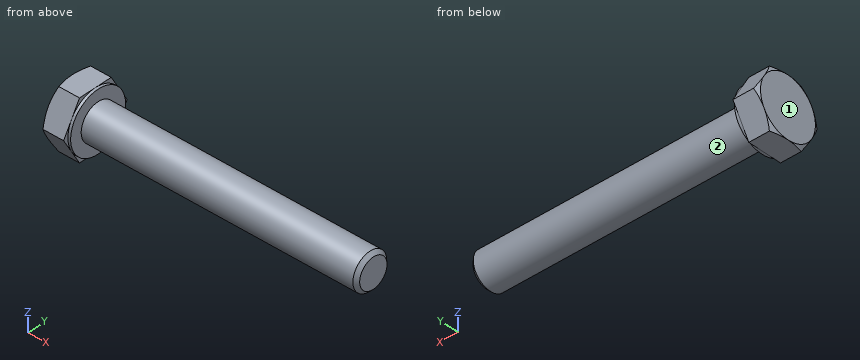
Autodesk Inventor part; units mm, degrees
ref_plane "Work Plane1" through (1.525, 0, 0) normal (0, 0, 1) x (1, 0, 0)
ref_plane "YZ Plane" through (0, 0, 0) normal (1, 0, 0) x (0, 1, 0)
ref_plane "XZ Plane" through (0, 0, 0) normal (0, 1, 0) x (-1, 0, 0)
sketch "Sketch1" plane through (0, 0, 0) normal (0, 0, 1) x (1, 0, 0)
  line L0 (0, 6.5) -> (0, 4)
  line L1 (38, 4) -> (60, 4)
  line L2 (60, 4) -> (60, 0)
  line L3 (60, 0) -> (-0.6001, 0)
  line L4 (-12.7201, 0) -> (72.12, 0)
  line L5 (-0.6001, 0) -> (-0.6001, 6.5)
  line L6 (-0.6001, 6.5) -> (0, 6.5)
  line L7 (38, 4) -> (37.2331, 4)
  line L8 (37.2331, 4) -> (0, 4)
  line L9 (0, -1.3) -> (0, 7.8)
  dimension "d0" = 60
  dimension "d1" = 22
  dimension "d2" = 8
  dimension "d9" = 0.6001
  dimension "d10" = 13
  dimension "d13" = 0.7669
  dimension "d14" = 8
revolve "Body" add sketch "Sketch1" angle 360 about axis through (60, 0, 0) along (-1, 0, 0)
sketch "Sketch2" plane through (-0.6001, 0, 0) normal (-1, 0, 0) x (0, 0, 1)
  line L0 (0, 7.5056) -> (6.5, 3.7528)
  line L1 (6.5, 3.7528) -> (6.5, -3.7528)
  line L2 (6.5, -3.7528) -> (0, -7.5056)
  line L3 (0, -7.5056) -> (-6.5, -3.7528)
  line L4 (-6.5, -3.7528) -> (-6.5, 3.7528)
  line L5 (-6.5, 3.7528) -> (0, 7.5056)
  point P0 (0, 0)
  point P1 (0, 0)
  dimension "d11" = 13
extrude "Head" add sketch "Sketch2" along normal blind 5.08
sketch "Sketch4" plane through (0, 0, 0) normal (0, 0, 1) x (1, 0, 0)
  line L0 (-5.6801, 6.5) -> (-5.6801, 7.5056)
  line L1 (-5.6801, 7.5056) -> (-5.0995, 7.5056)
  line L2 (-5.0995, 7.5056) -> (-5.6801, 6.5)
  line L3 (-6.6961, 0) -> (0.4159, 0)
  line L4 (-0.6001, 7.5056) -> (-5.6801, 7.5056)
  line L5 (-5.6801, 3.7528) -> (-5.6801, 7.5056)
  dimension "d5" = 30
  dimension "d19" = 13
revolve "Chamfer1" cut sketch "Sketch4" angle 360 about axis through (-10, 0, 0) along (1, 0, 0)
thread "Thread"
chamfer "Chamfer2" distance 0.7668 distance2 0.7669 1 edges at (60, -4, 0) measured on face at (60, -0.1514, -1.2467)
ref_plane "Work Plane1" through (1.525, 0, 0) normal (0, 0, 1) x (1, 0, 0)
equation "\"d0\" = NLG"
equation "\"d1\" = GEL"
equation "\"d2\" = GD"
equation "\"d10\" = SD2"
equation "\"d14\" = BDM"
equation "\"d11\" = SW"
equation "\"d3\" = KOH - SD"
equation "\"d5\" = ANG1"
equation "\"d19\" = SW0"
equation "\"d15\" = GEL"
equation "\"d6\" = -0.5 * SPD + 0.5 * GD"
equation "\"NLG\" = 60"
equation "\"GD\" = NND"
equation "\"BDM\" = NND"
equation "\"KOH\" = 5.68"
equation "\"GEL\" = 22"
equation "\"SW\" = 13"
equation "\"SW0\" = SW"
equation "\"SPD\" = NND - 1.2269 * PTC"
equation "\"SD2\" = SW"
equation "\"SD\" = 0.6"
equation "\"ANG1\" = 30deg"
equation "\"GAL\" = 0.61345 * PTC"
equation "\"GUL\" = 0.61345 * PTC"
equation "\"RR\" = 0.4"
equation "\"WFT\" = SD"
equation "\"GD1\" = THREADDIA - 1.2269 * PTC"
equation "\"THREADDIA\" = 8"
equation "\"SDH\" = SW"
equation "\"TOA\" = 30deg"
equation "\"FAWI\" = 45deg"
equation "\"PTC\" = 1.25"
equation "\"NND\" = 8"
equation "\"E0\" = 1.155 * SW"
properties part number "AS 1111 - M8 x 60" material "Steel, Mild"
Model file for the job. Use its own axes, mm. Face numbers are marked on the shaded views. A direction names the side the tool comes from. Give positions to 0.01 mm unless a question says otherwise; leave off trailing zeros. Loops run counter-clockwise (first coordinate to the right, second up) from the corner with the lowest first, then second, coordinate; pieces in that order, holes last. Notation, with made-up numbers: (-3, -12.75) -> (55, -12.75) arc R26 cw to (55, 12.25) -> close; hole circle Ø8 at (41, -14). An arc over 180 degrees is marked (long way). Use CSV: the item, a comma, the result in double quotes. Start each with the question number.
1) Flat gauge pins, fed straight in: pin 1 Ø4 at (x, y) = (14, 3) entering from +Z; pin 2 Ø2 at (y, z) = (-6, -3.5) entering from +X; pin 3 Ø2.5 at (y, z) = (-5, 0) entering from +X. Where does each tip first touch, or does it go through?
2) Wall check: line 1 (X direction, y = 2.25, z = -4.5); line 2 (Y direction, x = 1.5, z = -0.25); line 3 (Z direction, x = 51, y = 0). Give the ranges that are in metal, low to high.
3) Tool access for the marked faces 1 and 2: list every direction of +Z, -Z, +X, -X, +Y, -Y with a clear straight run to the whole face (end or side of a thin tool).
4) Slice it at A-A on x = 43. Give the cut face in (y, z), plus the area to 3 significant figures.
Computed values:
1,pin 1,"stops at z = 3.87"
1,pin 2,"stops at x = 0"
1,pin 3,"stops at x = 59.48"
2,line 1,"x = -5.68 to 0"
2,line 2,"y = -3.99 to 3.99"
2,line 3,"z = -4 to 4"
3,face 1,"+Z, -Z, -X, +Y, -Y"
3,face 2,"+X"
4,outline,"circle Ø8 at (0, 0)"
4,area,"50.3 mm^2"
